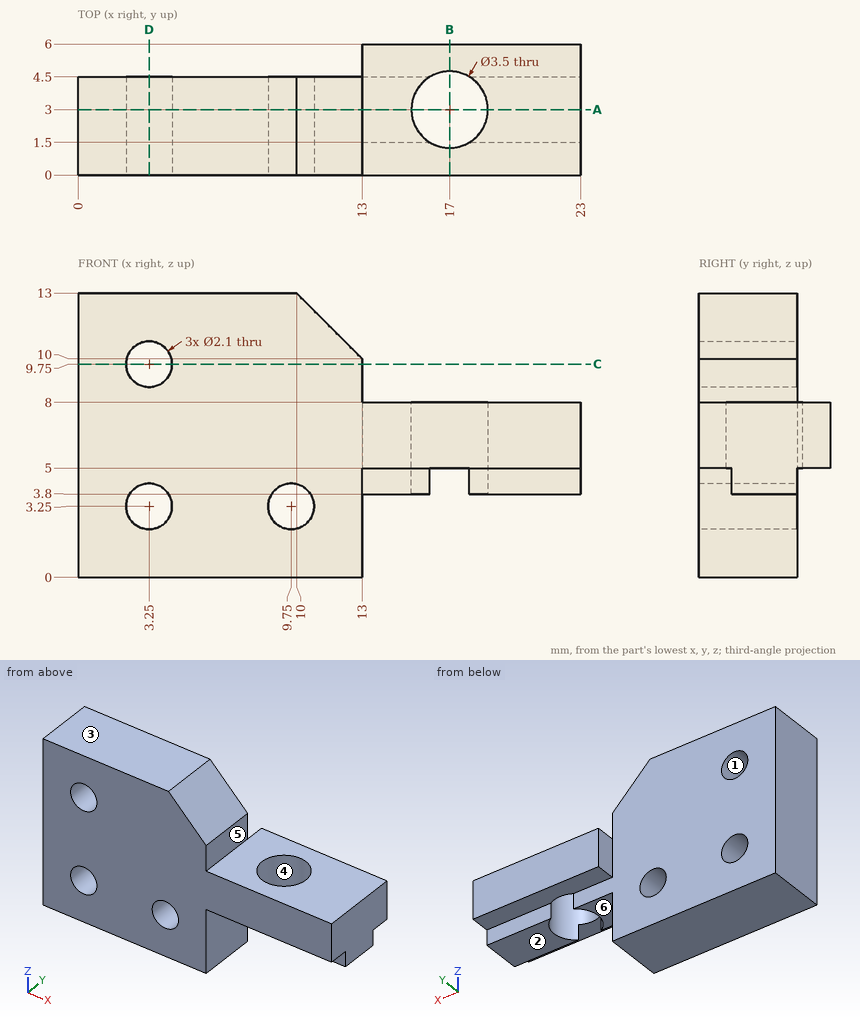
Geometry: see drawing. Coordinates: mm, zero at the bounding-box minimum. A direction names the side the tool comes from. Round coordinates to 2 decimals unless told otherwise and drop trailing zeros. Write each loop counter-clockwise with the first axis right and the second up, starting at its lowest first coordinate (ties: lowest second). Pieces come first, ordered by that corner, then holes. Notation, with made-up numbers: M 69.5,11.25 L 115.5,11.25 A20 ccw 115.5,49.25 Z; hole C 3,-27 d5. An arc over 180 degrees is marked long. Answer in a Markdown table with one row per item. Add a question column.
(1) Contact query for flat-ended pins moving along their axis: pin 1 (0.6 mm diameter, centred on y = 2.5, z = 9, fed in from +X); pin 2 (2.5 mm diameter, centred on x = 20.5, y = 2.5, fed in from -Z); pin 3 (1.5 mm diameter, centred on x = 14.5, y = 2, fed in from +Z). Output: stop coordinate, or through.
(2) Cut plane B-B, the plane x = 17. Return the cut outline in (y, z).
(3) Cut plane A-A, the plane y = 3. Return the cut outline in (x, z), then the cut area to 3 significant figures.
(4) Ray query, L1, parallel to X at y = 1, z = 3.25; L2, parallel to X at y = 2.75, z = 2.75. Return the intervals inside material, ascending.
(5) Reachability of the marked faces 4, 5 and 6 from +Z, -Z, +X, -X, +Y, -Y: full face, straight path, thin tool, end or side. Return the list, or none.
(6) Cut plane D-D, the plane x = 3.25. Return the cut outline in (y, z), then the cut area to 3 significant figures.
(7) Draft query along Z for the marked faces 1, 2 and 3. Return one class per face: pulls with the +Z half, pulls with the -Z half, needs draft (parallel to the pull), parting line crosses it, or undercut.
(8) Cut plane C-C, the plane z = 9.75. Return the cut outline in (x, y).
Established:
| question | item | result |
|---|---|---|
| 1 | pin 1 | x = 13 |
| 1 | pin 2 | z = 3.8 |
| 1 | pin 3 | z = 8 |
| 2 | outline | M 0,5 L 1.25,5 L 1.25,8 L 0,8 Z; M 4.75,5 L 6,5 L 6,8 L 4.75,8 Z |
| 3 | outline | M 0,0 L 13,0 L 13,3.8 L 15.25,3.8 L 15.25,8 L 13,8 L 13,10 L 10,13 L 0,13 Z; M 18.75,3.8 L 23,3.8 L 23,8 L 18.75,8 Z; hole C 3.25,3.25 d2.1; hole C 3.25,9.75 d2.1; hole C 9.75,3.25 d2.1 |
| 3 | area | 181 mm² |
| 4 | L1 | 0 to 2.2, 4.3 to 8.7, 10.8 to 13 |
| 4 | L2 | 0 to 2.33, 4.17 to 8.83, 10.67 to 13 |
| 5 | face 4 | +Z, -Z |
| 5 | face 5 | +Z, +X, +Y, -Y |
| 5 | face 6 | -Z, +X, +Y, -Y |
| 6 | outline | M 0,0 L 4.5,0 L 4.5,2.2 L 0,2.2 Z; M 0,4.3 L 4.5,4.3 L 4.5,8.7 L 0,8.7 Z; M 0,10.8 L 4.5,10.8 L 4.5,13 L 0,13 Z |
| 6 | area | 39.6 mm² |
| 7 | face 1 | undercut |
| 7 | face 2 | pulls with the -Z half |
| 7 | face 3 | pulls with the +Z half |
| 8 | outline | M 0,0 L 2.2,0 L 2.2,4.5 L 0,4.5 Z; M 4.3,0 L 13,0 L 13,4.5 L 4.3,4.5 Z |
